Autodesk Inventor part; units mm, degrees
ref_plane "YZ Plane" through (0, 0, 0) normal (1, 0, 0) x (0, 1, 0)
ref_plane "XZ Plane" through (0, 0, 0) normal (0, 1, 0) x (-1, 0, 0)
ref_plane "XY Plane" through (0, 0, 0) normal (0, 0, 1) x (1, 0, 0)
sketch "草图1" plane through (0, 0, 0) normal (0, 0, 1) x (1, 0, 0)
  circle A0 centre (0, 0) radius 4.5
  dimension "d0" = 9
extrude "拉伸1" add sketch "草图1" along normal blind 1
sketch "草图2" plane through (0, 0, 1) normal (0, 0, 1) x (1, 0, 0)
  line L0 (1.8764, -3.25) -> (-1.8764, -3.25)
  line L1 (-1.8764, -3.25) -> (-3.7528, 0)
  line L2 (-3.7528, 0) -> (-1.8764, 3.25)
  line L3 (-1.8764, 3.25) -> (1.8764, 3.25)
  line L4 (1.8764, 3.25) -> (3.7528, 0)
  line L5 (3.7528, 0) -> (1.8764, -3.25)
  line L6 (0, 0) -> (0, 3.25)
  dimension "d3" = 6.5
extrude "拉伸2" add sketch "草图2" along normal blind 4
sketch "草图3" plane through (0, 0, 5) normal (0, 0, 1) x (1, 0, 0)
  circle A0 centre (0, 0) radius 2.5
  dimension "d6" = 5
extrude "拉伸3" cut sketch "草图3" against normal through all
thread "螺纹1"
properties part number "刮肉轮固定螺丝"
Read the model definition and answer for the solid it produces. Units are mm, in the model's axes. A direction names the side the tool comes from. Coordinates: 2 decimals unless noted, no trailing zeros. Write each loop counter-clockwise with the first axis right and the second up, starting at its lowest first coordinate (ties: lowest second). Pieces come first, ordered by that corner, then holes. Notation, with made-up numbers: (75, 35) - (97, 35) arc R6 cw to (97, 42) - close; hole circle Ø8 at (21.25, 39). An arc over 180 degrees is marked (long way). Answer as a JSON object with one key per item and string values. Group by question number.
1. Which of the six approach directions +Z, -Z, +X, -X, +Y, -Y give full straight-line access (tool end or side, diameter ignored) to faces 4 (the flat face through (2.8, 1.65, 2.97)), 5 (the flat face through (0, 3.25, 3)), 6 (the flat face through (-2.8, -1.65, 2.97))?
2. A cutting plane is placed at B-B (z = 2.35). Determine the outline of the cut face in (x, y).
3. The mould has two halves that part along Y. Classify faces 1 (the cylindrical face through (-0.54, -2.44, 2.54)), 2 (the flat face through (-2.83, 1.6, 2.97)), 3 (the flat face through (2.83, -1.6, 2.97)): +Y half, -Y half, draft (parallel to the pull), parting line (faces both ways), or undercut.
4. Each of these flat-tipped pins is pushed along its axis until it touches: P1, Ø1.9, axis at x = -1, z = 3, coming from the -Y side; P2, Ø2, axis at x = 3.5, z = 3.5, coming from the -Y side. Where does it stop, or does it pass through?
5. A cutting plane is placed at C-C (y = -0.5). Determine the outline of the cut face in (x, z), plus the area to 3 significant figures.
6. A cutting plane is placed at A-A (x = 0). Determine the outline of the cut face in (y, z).
7. A cutting plane is placed at D-D (x = 3). Determine the outline of the cut face in (y, z), plus the area to 3 significant figures.
8. Consider L1, parallel to Y at x = 0, z = 3.45; L2, parallel to Z at x = 3.25, y = 1.75; L3, parallel to X at y = -1.5, z = 2.5. Determine where each line is inside the solid, lowest interval first. Write a range as [from, to].
Worked out:
{
 "1": {"face 4": "+Z, +X, +Y", "face 5": "+Z, +X, -X, +Y", "face 6": "+Z, -X, -Y"},
 "2": {"outline": "(-3.75, 0) - (-1.88, -3.25) - (1.88, -3.25) - (3.75, 0) - (1.88, 3.25) - (-1.88, 3.25) - close; hole circle Ø5 at (0, 0)"},
 "3": {"face 1": "undercut", "face 2": "+Y half", "face 3": "-Y half"},
 "4": {"P1": "stops at y = -3.25", "P2": "stops at y = -2.17"},
 "5": {"outline": "(-4.47, 0) - (-2.45, 0) - (-2.45, 5) - (-3.46, 5) - (-3.46, 1) - (-4.47, 1) - close; (2.45, 0) - (4.47, 0) - (4.47, 1) - (3.46, 1) - (3.46, 5) - (2.45, 5) - close", "area": "12.2 mm²"},
 "6": {"outline": "(-4.5, 0) - (-2.5, 0) - (-2.5, 5) - (-3.25, 5) - (-3.25, 1) - (-4.5, 1) - close; (2.5, 0) - (4.5, 0) - (4.5, 1) - (3.25, 1) - (3.25, 5) - (2.5, 5) - close"},
 "7": {"outline": "(-3.35, 0) - (3.35, 0) - (3.35, 1) - (1.3, 1) - (1.3, 5) - (-1.3, 5) - (-1.3, 1) - (-3.35, 1) - close", "area": "17.1 mm²"},
 "8": {"L1": "y = [-3.25, -2.5], [2.5, 3.25]", "L2": "z = [0, 1]", "L3": "x = [-2.89, -2], [2, 2.89]"}
}
